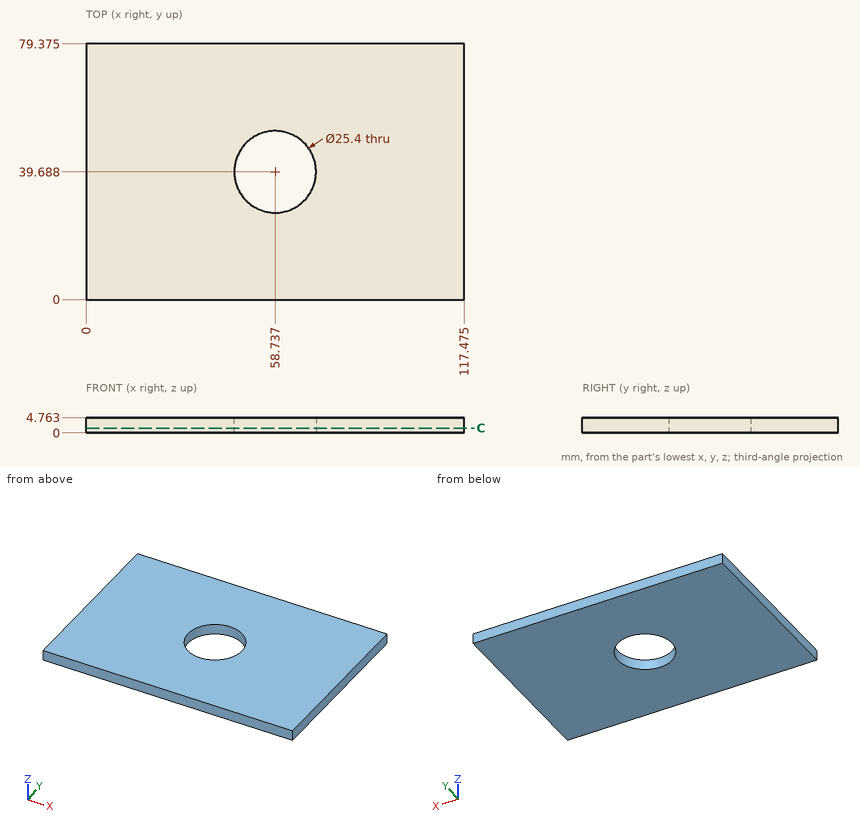
The figure shows three views and two pictorial views of one solid part (mm, origin at its lowest corner). Answer the questions. Give positions to 0.01 mm unless a question says otherwise; leave off trailing zeros. Loops run counter-clockwise (first coordinate to the right, second up) from the corner with the lowest first, then second, coordinate; pieces in that order, holes last. Notation, with made-up numbers: (-10, 74.25) -> (17, 74.25) arc R19 ccw to (17, 107.25) -> close; hole circle Ø8 at (36.25, 52.25). An arc over 180 degrees is marked (long way). Use a Markdown table: item, result. Add a question column.
1. Section C-C on z = 1.5 is taken. Determine the outline of the cut face in (x, y) (1 decimal).
2. Find the intervals of material crossed by probe 1 along X at (y, z) = (39, 3.8) (1 decimal); probe 2 along X at (y, z) = (33.5, 3.5) (1 decimal); probe 3 along Y at (x, z) = (54.5, 3.45) (1 decimal), in increasing order.
3. Flat-ended cylindrical pins translate along their axes: pin 1 Ø4 at (x, y) = (57.5, 29) entering from -Z; pin 2 Ø20.5 at (x, y) = (58.74, 39.69) entering from -Z. Find the tip coordinate at first contact, or state that the pin passes through.
Results below:
| question | item | result |
|---|---|---|
| 1 | outline | (0, 0) -> (117.5, 0) -> (117.5, 79.4) -> (0, 79.4) -> close; hole circle Ø25.4 at (58.7, 39.7) |
| 2 | probe 1 | x = 0 to 46.1, 71.4 to 117.5 |
| 2 | probe 2 | x = 0 to 47.6, 69.8 to 117.5 |
| 2 | probe 3 | y = 0 to 27.7, 51.7 to 79.4 |
| 3 | pin 1 | stops at z = 0 |
| 3 | pin 2 | passes through |
